```python
from build123d import *

# Parameters (mm, degrees)
SALIENTE_EXTRUIR1_DEPTH = 432
CORTAR_EXTRUIR1_DEPTH   = 433.072331908
CORTAR_EXTRUIR2_DEPTH   = 433.072331908
CORTAR_EXTRUIR3_DEPTH   = 433.072331908
CORTAR_EXTRUIR4_DEPTH   = 433.072331908
CORTAR_EXTRUIR5_DEPTH   = 433.072331908
CORTAR_EXTRUIR6_DEPTH   = 433.072331908
CORTAR_EXTRUIR7_DEPTH   = 0.002166667
CORTAR_EXTRUIR8_DEPTH   = 0.002166667
CORTAR_EXTRUIR9_DEPTH   = 0.002166667
CORTAR_EXTRUIR10_DEPTH  = 0.002166667
NGULO_DE_SALIDA1_ANGLE  = 45.1469538
CHAFL_N1_SIZE           = 0.4
REDONDEO1_R             = 0.130000023
MATRIZL2_COUNT          = 21
MATRIZL2_PITCH          = 20


with BuildPart() as part:
    # Croquis1 → Saliente-Extruir1 (new body)
    with BuildSketch(Plane.XZ):
        Polygon((4.5, 0), (4.5, 6.01167813), (4.1, 6.50000002), (-4.1, 6.50000002), (-4.5, 6.01167813), (-4.5, 0), align=None)
    extrude(amount=-SALIENTE_EXTRUIR1_DEPTH)

    # Croquis2 → Cortar-Extruir1 (cut, through all)
    with BuildSketch(Plane(origin=(0, 432, 0), x_dir=(-1, 0, 0), z_dir=(0, 1, 0))):
        with BuildLine():
            Line((-4.5, 4.88017535), (-4.5, 4.03150278))
            Line((-4.5, 4.03150278), (-3.819258765, 4.03150278))
            ThreePointArc((-3.819258765, 4.03150278), (-3.21946318, 4.455839065), (-3.819258765, 4.88017535))
            Line((-3.819258765, 4.88017535), (-4.5, 4.88017535))
        make_face()
    extrude(amount=-CORTAR_EXTRUIR1_DEPTH, mode=Mode.SUBTRACT)

    # Croquis3 → Cortar-Extruir2 (cut, through all)
    with BuildSketch(Plane(origin=(0, 432, 0), x_dir=(-1, 0, 0), z_dir=(0, 1, 0))):
        with BuildLine():
            Line((-4.026513856, 4.03150278), (-4.5, 4.03150278))
            Line((-4.5, 4.03150278), (-4.5, 3.583620931))
            ThreePointArc((-4.5, 3.583620931), (-4.223645982, 3.76568645), (-4.026513856, 4.03150278))
        make_face()
    extrude(amount=-CORTAR_EXTRUIR2_DEPTH, mode=Mode.SUBTRACT)

    # Croquis4 → Cortar-Extruir3 (cut, through all)
    with BuildSketch(Plane(origin=(0, 432, 0), x_dir=(-1, 0, 0), z_dir=(0, 1, 0))):
        with BuildLine():
            Line((-4.5, 5.328056964), (-4.5, 4.88017535))
            Line((-4.5, 4.88017535), (-4.026513974, 4.88017535))
            ThreePointArc((-4.026513974, 4.88017535), (-4.223646078, 5.145991535), (-4.5, 5.328056964))
        make_face()
    extrude(amount=-CORTAR_EXTRUIR3_DEPTH, mode=Mode.SUBTRACT)

    # Croquis5 → Cortar-Extruir4 (cut, through all)
    with BuildSketch(Plane(origin=(0, 432, 0), x_dir=(-1, 0, 0), z_dir=(0, 1, 0))):
        with BuildLine():
            Line((4.5, 4.03150278), (4.5, 4.88017535))
            Line((4.5, 4.88017535), (3.819258765, 4.88017535))
            ThreePointArc((3.819258765, 4.88017535), (3.21946318, 4.455839065), (3.819258765, 4.03150278))
            Line((3.819258765, 4.03150278), (4.5, 4.03150278))
        make_face()
    extrude(amount=-CORTAR_EXTRUIR4_DEPTH, mode=Mode.SUBTRACT)

    # Croquis6 → Cortar-Extruir5 (cut, through all)
    with BuildSketch(Plane(origin=(0, 432, 0), x_dir=(-1, 0, 0), z_dir=(0, 1, 0))):
        with BuildLine():
            Line((4.026513826, 4.88017535), (4.5, 4.88017535))
            Line((4.5, 4.88017535), (4.5, 5.328057255))
            ThreePointArc((4.5, 5.328057255), (4.223645966, 5.145991706), (4.026513826, 4.88017535))
        make_face()
    extrude(amount=-CORTAR_EXTRUIR5_DEPTH, mode=Mode.SUBTRACT)

    # Croquis7 → Cortar-Extruir6 (cut, through all)
    with BuildSketch(Plane(origin=(0, 432, 0), x_dir=(-1, 0, 0), z_dir=(0, 1, 0))):
        with BuildLine():
            Line((4.5, 3.583620926), (4.5, 4.03150278))
            Line((4.5, 4.03150278), (4.026513851, 4.03150278))
            ThreePointArc((4.026513851, 4.03150278), (4.223645987, 3.765686455), (4.5, 3.583620926))
        make_face()
    extrude(amount=-CORTAR_EXTRUIR6_DEPTH, mode=Mode.SUBTRACT)

    # Croquis8 → Cortar-Extruir7 (cut)
    with BuildSketch(Plane(origin=(0, 432, 0), x_dir=(-1, 0, 0), z_dir=(0, 1, 0))):
        Polygon((0.891369267, 3.403698133), (0.714701433, 3.168235633), (0.2187042, 2.61105), (1.0945792, 2.61105), (1.0945792, 2.695983333), (0.398689633, 2.695983333), (0.794326433, 3.149466667), (0.9743123, 3.3891), (1.067110588, 3.573407857), (0.95413722, 3.802321701), (0.7876908, 3.88505), (0.54301, 3.88505), (0.375434678, 3.803592619), (0.295011167, 3.6384023), (0.295011167, 3.562), (0.3812718, 3.562), (0.3812718, 3.631766667), (0.437672733, 3.743620833), (0.549645633, 3.800116667), (0.7802262, 3.800116667), (0.893028067, 3.743810633), (0.976240026, 3.576039029), align=None)
    extrude(amount=-CORTAR_EXTRUIR7_DEPTH, mode=Mode.SUBTRACT)

    # Croquis9 → Cortar-Extruir8 (cut)
    with BuildSketch(Plane.XZ):
        Polygon((-0.214632167, 3.88505), (-0.953983333, 3.88505), (-0.953983333, 2.61105), (-0.214632167, 2.61105), (-0.214632167, 2.695983333), (-0.86905, 2.695983333), (-0.86905, 3.205583333), (-0.5123963, 3.205583333), (-0.5123963, 3.290516667), (-0.86905, 3.290516667), (-0.86905, 3.800116667), (-0.214632167, 3.800116667), align=None)
    extrude(amount=-CORTAR_EXTRUIR8_DEPTH, mode=Mode.SUBTRACT)

    # Croquis10 → Cortar-Extruir9 (cut)
    with BuildSketch(Plane(origin=(0, 432, 0), x_dir=(-1, 0, 0), z_dir=(0, 1, 0))):
        Polygon((-0.214632167, 3.88505), (-0.953983333, 3.88505), (-0.953983333, 2.61105), (-0.214632167, 2.61105), (-0.214632167, 2.695983333), (-0.86905, 2.695983333), (-0.86905, 3.205583333), (-0.5123963, 3.205583333), (-0.5123963, 3.290516667), (-0.86905, 3.290516667), (-0.86905, 3.800116667), (-0.214632167, 3.800116667), align=None)
    extrude(amount=-CORTAR_EXTRUIR9_DEPTH, mode=Mode.SUBTRACT)

    # Croquis11 → Cortar-Extruir10 (cut)
    with BuildSketch(Plane.XZ):
        Polygon((0.510057167, 3.620830633), (0.6071, 3.718655633), (0.6071, 2.609403333), (0.692033333, 2.609403333), (0.692033333, 3.883403333), (0.6741176, 3.883403333), (0.6741176, 3.795069794), (0.3690544, 3.640736667), (0.3690544, 3.551253333), align=None)
    extrude(amount=-CORTAR_EXTRUIR10_DEPTH, mode=Mode.SUBTRACT)

    # Ángulo de salida1
    ngulo_de_salida1_faces = [part.faces().sort_by_distance(p)[0] for p in [
        (0.6741176, 0.001083333, 3.839236564),
    ]]
    draft(ngulo_de_salida1_faces, Plane(origin=(0.692033333, 0.002166667, 3.883403333), x_dir=(-1, 0, 0), z_dir=(0, 0, -1)), NGULO_DE_SALIDA1_ANGLE)

    # Chaflán1
    chafl_n1_edges = [part.edges().sort_by_distance(p)[0] for p in [
        (-4.5, 216, 0),
        (4.5, 216, 0),
    ]]
    chamfer(chafl_n1_edges, length=CHAFL_N1_SIZE)

    # Redondeo1
    redondeo1_edges = [part.edges().sort_by_distance(p)[0] for p in [
        (4.026513856, 216, 4.03150278),
        (4.5, 216, 3.583620931),
        (4.5, 216, 5.328056964),
        (4.026513974, 216, 4.88017535),
        (-4.026513826, 216, 4.88017535),
        (-4.5, 216, 5.328057255),
        (-4.5, 216, 3.583620926),
        (-4.026513851, 216, 4.03150278),
    ]]
    fillet(redondeo1_edges, radius=REDONDEO1_R)

    # Croquis34 → Taladro roscado M3.5x0.61 (revolve, cut)
    with BuildSketch(Plane(origin=(0, 16, 0), x_dir=(0, 1, 0), z_dir=(1, 0, 0))):
        Polygon((0, 0), (0, 8), (3, 8), (3, 3), (1.75, 3), (1.75, 0), align=None)
    taladro_roscado_m3_5x0_61 = revolve(axis=Axis((0, 16, -6.35), (0, 0, 1)), mode=Mode.SUBTRACT)

    # MatrizL2: Taladro roscado M3.5x0.61 ×21
    with Locations(*[(0, i * MATRIZL2_PITCH, 0) for i in range(1, MATRIZL2_COUNT)]):
        add(taladro_roscado_m3_5x0_61, mode=Mode.SUBTRACT)


solid = part.part
```
Here's how the part is built. I have some questions about the finished solid (model axes, mm). Give positions to 0.01 mm unless a question says otherwise; leave off trailing zeros. Order: outer loops, then holes, each group sorted by start corner. A loop starts at its lowest first (then second) coordinate and runs counter-clockwise, first axis right, second up. Notation, with made-up numbers: M 11,62.25 L 32,62.25 A8 ccw 32,70.25 Z; hole C 85,78 d9. An arc over 180 degrees is marked long. Use a Markdown table: item, result. Add a question column.
1. For pin 1 Ø4.5 at (x, y) = (0, 376) entering from +Z; pin 2 Ø4.5 at (x, y) = (0, 256) entering from -Z; pin 3 Ø2 at (x, y) = (0, 336) entering from +Z, each with a flat end and sliding along its axis, tell me the tip position at first contact or that it passes through.
2. Suppose I cut it at A-A (y = 105.5). List the corners of the cut face in (x, z) for me.
3. I need wall thicknesses on probe 1 along Z at (x, y) = (3.5, 109.5); probe 2 along X at (y, z) = (396, 2.2); probe 3 along X at (y, z) = (116, 5.5). Which ranges of each line are inside material? Lowest first, please. Write a range as from..to.
Results list:
| question | item | result |
|---|---|---|
| 1 | pin 1 | stops at z = 3 |
| 1 | pin 2 | stops at z = 0 |
| 1 | pin 3 | passes through |
| 2 | outline | M -4.5,0.4 L -4.1,0 L 4.1,0 L 4.5,0.4 L 4.5,3.5 A0.13 ccw 4.43,3.62 A0.95 cw 4.06,3.97 A0.13 ccw 3.95,4.03 L 3.82,4.03 A0.45 cw long 3.82,4.88 L 3.95,4.88 A0.13 ccw 4.06,4.94 A0.95 cw 4.43,5.29 A0.13 ccw 4.5,5.41 L 4.5,6.01 L 4.1,6.5 L -4.1,6.5 L -4.5,6.01 L -4.5,5.41 A0.13 ccw -4.43,5.29 A0.95 cw -4.06,4.94 A0.13 ccw -3.95,4.88 L -3.82,4.88 A0.45 cw long -3.82,4.03 L -3.95,4.03 A0.13 ccw -4.06,3.97 A0.95 cw -4.43,3.62 A0.13 ccw -4.5,3.5 Z |
| 3 | probe 1 | z = 0..4.04, 4.87..6.5 |
| 3 | probe 2 | x = -4.5..-1.75, 1.75..4.5 |
| 3 | probe 3 | x = -4.5..-3, 3..4.5 |
